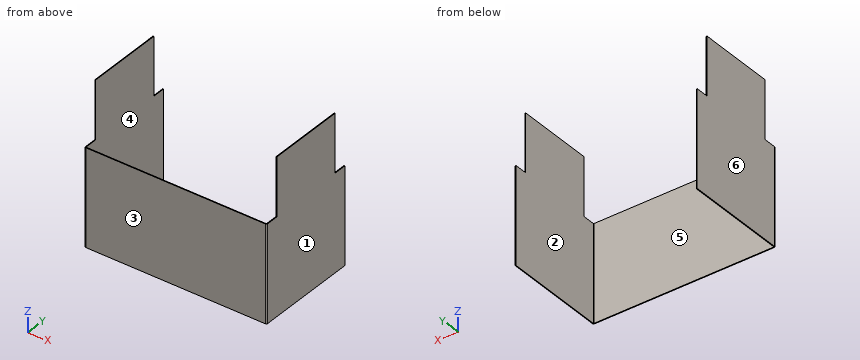
from build123d import *

# Parameters (mm, degrees)
SKETCH1_W                      = 317.5
SKETCH1_H                      = 1.5875
BASE_FLANGE1_DEPTH             = 355.6
EDGE_FLANGE1_STRIP_W           = 7.8232
EDGE_FLANGE1_STRIP_H           = 1.5875
EDGE_FLANGE1_STRIP_CUT_DEPTH   = 317.5
EDGE_FLANGE1_STRIP_2_W         = 7.8232
EDGE_FLANGE1_STRIP_2_H         = 1.5875
EDGE_FLANGE1_STRIP_CUT_2_DEPTH = 317.5
EDGE_FLANGE1_DEPTH             = 317.5
EDGE_FLANGE1_BEND_DEPTH        = 317.5
SKETCH8_W                      = 114.3
SKETCH8_H                      = 152.4
BOSS_EXTRUDE1_DEPTH            = 1.5875
SKETCH10_W                     = 127
SKETCH10_H                     = 254
CUT_EXTRUDE1_DEPTH             = 598.585693253


# Sheet-metal steps are written as plain solids
with BuildPart() as part:
    # Sketch1 → Base-Flange1 (new body)
    with BuildSketch(Plane(origin=(0, 0, 0), x_dir=(0, 0, -1), z_dir=(1, 0, 0))):
        with Locations((-158.75, 0.79375)):
            Rectangle(SKETCH1_W, SKETCH1_H)
    extrude(amount=BASE_FLANGE1_DEPTH)

    # Edge-Flange1 strip (across the edge) → Edge-Flange1 strip cut (cut)
    with BuildSketch(Plane(origin=(355.6, 1.5875, 317.5), x_dir=(-1, 0, 0), z_dir=(0, 0, -1))):
        with Locations((-3.175, -0.79375)):
            Rectangle(EDGE_FLANGE1_STRIP_W, EDGE_FLANGE1_STRIP_H)
    extrude(amount=EDGE_FLANGE1_STRIP_CUT_DEPTH, mode=Mode.SUBTRACT)

    # Edge-Flange1 strip 2 (across the edge) → Edge-Flange1 strip cut 2 (cut)
    with BuildSketch(Plane(origin=(0, 1.5875, 0), x_dir=(1, 0, 0), z_dir=(0, 0, 1))):
        with Locations((-3.175, -0.79375)):
            Rectangle(EDGE_FLANGE1_STRIP_2_W, EDGE_FLANGE1_STRIP_2_H)
    extrude(amount=EDGE_FLANGE1_STRIP_CUT_2_DEPTH, mode=Mode.SUBTRACT)

    # Edge-Flange1 section (across the edge) → Edge-Flange1 (add)
    with BuildSketch(Plane(origin=(355.6, 1.5875, 317.5), x_dir=(-1, 0, 0), z_dir=(0, 0, -1))):
        with BuildLine():
            Line((-1.5875, 0.7366), (-1.5875, 203.2))
            Line((-1.5875, 203.2), (0, 203.2))
            Line((0, 203.2), (0, 0.7366))
            ThreePointArc((0, 0.7366), (0.215745145, 0.215745145), (0.7366, 0))
            Line((0.7366, 0), (0.7366, -1.5875))
            ThreePointArc((0.7366, -1.5875), (-0.90678687, -0.90678687), (-1.5875, 0.7366))
        make_face()
    extrude(amount=EDGE_FLANGE1_DEPTH)

    # Edge-Flange1 section 2 (across the edge) → Edge-Flange1 bend (add)
    with BuildSketch(Plane(origin=(0, 1.5875, 0), x_dir=(1, 0, 0), z_dir=(0, 0, 1))):
        with BuildLine():
            Line((-1.5875, 0.7366), (-1.5875, 203.2))
            Line((-1.5875, 203.2), (0, 203.2))
            Line((0, 203.2), (0, 0.7366))
            ThreePointArc((0, 0.7366), (0.215745145, 0.215745145), (0.7366, 0))
            Line((0.7366, 0), (0.7366, -1.5875))
            ThreePointArc((0.7366, -1.5875), (-0.90678687, -0.90678687), (-1.5875, 0.7366))
        make_face()
    extrude(amount=EDGE_FLANGE1_BEND_DEPTH)


with BuildPart() as body_2:
    # Sketch8 → Boss-Extrude1 (new body)
    with BuildSketch(Plane(origin=(357.1875, 0, 0), x_dir=(0, 0, -1), z_dir=(1, 0, 0))):
        with Locations((-374.65, 103.1875)):
            Rectangle(SKETCH8_W, SKETCH8_H)
    extrude(amount=-BOSS_EXTRUDE1_DEPTH)


with BuildPart() as body_3:
    # Mirror1: mirrored copy
    add(body_2.part.mirror(Plane(origin=(177.8, 0, 0), x_dir=(0, 0, 1), z_dir=(1, 0, 0))))


with BuildPart() as body_2_1:
    add(body_2.part)

    # Combine1: union part, body 3
    add(part.part)
    add(body_3.part)

    # Sketch10 → Cut-Extrude1 (cut, through all)
    with BuildSketch(Plane(origin=(357.1875, 0, 0), x_dir=(0, 0, -1), z_dir=(1, 0, 0))):
        with Locations((-63.5, 77.7875)):
            Rectangle(SKETCH10_W, SKETCH10_H)
    extrude(amount=-CUT_EXTRUDE1_DEPTH, mode=Mode.SUBTRACT)


solid = body_2_1.part
Verification items for the finished model (mm, model axes). Face numbers are marked on the shaded views. A direction names the side the tool comes from. Coordinates: 2 decimals unless noted, no trailing zeros. Order: outer loops, then holes, each group sorted by start corner. A loop starts at its lowest first (then second) coordinate and runs counter-clockwise, first axis right, second up.
Item 1: Depth check by flat-ended pin: pin 1 (21.5 mm diameter, centred on x = 181.5, y = 13, fed in from +Z); pin 2 (1 mm diameter, centred on x = 241.5, z = 238, fed in from +Y); pin 3 (1.7 mm diameter, centred on x = -0.5, z = 374.5, fed in from +Y); pin 4 (1.7 mm diameter, centred on x = 357, z = 370.5, fed in from -Y). Enter the tip coordinate at first touch or a pass-through.
Filled in:
pin 1: passes through
pin 2: stops at y = 1.59
pin 3: stops at y = 179.39
pin 4: stops at y = 26.99
Item 2: Release check for a two-part mould opening along X. For the marked faces 1, 2, 3 and 4 record: +X half, -X half, draft (parallel to the pull), parting line (faces both ways), or undercut.
Filled in:
face 1: +X half
face 2: undercut
face 3: draft
face 4: undercut
Item 3: Access from +Z, -Z, +X, -X, +Y, -Y to the whole of each face (thin tool, end or side, straight path). Record for the marked faces 5 and 6.
Filled in:
face 5: +Z, -Z, +Y
face 6: +Z, -Z, -X, +Y, -Y
Item 4: Section check C-C, the plane z = 291. Enter the section's corners in (x, y), then the cut area to 3 significant figures.
Filled in:
outline: (-1.59, 2.32) arc R2.32 ccw to (0.74, 0) - (354.86, 0) arc R2.32 ccw to (357.19, 2.32) - (357.19, 204.79) - (355.6, 204.79) - (355.6, 2.32) arc R0.74 cw to (354.86, 1.59) - (0.74, 1.59) arc R0.74 cw to (0, 2.32) - (0, 204.79) - (-1.59, 204.79) - close
area: 1,210 mm2
Item 5: Section check B-B, the plane y = 115.5. Enter the section's corners in (x, z).
Filled in:
outline: (-1.59, 127) - (0, 127) - (0, 431.8) - (-1.59, 431.8) - close; (355.6, 127) - (357.19, 127) - (357.19, 431.8) - (355.6, 431.8) - close
Item 6: Section check D-D, the plane x = 259.5. Enter the section's corners in (y, z), then the cut area to 3 significant figures.
Filled in:
outline: (0, 127) - (1.59, 127) - (1.59, 317.5) - (0, 317.5) - close
area: 302 mm2
Item 7: Section check A-A, the plane z = 406.5. Enter the section's corners in (x, y), then the cut area to 3 significant figures.
Filled in:
outline: (-1.59, 26.99) - (0, 26.99) - (0, 179.39) - (-1.59, 179.39) - close; (355.6, 26.99) - (357.19, 26.99) - (357.19, 179.39) - (355.6, 179.39) - close
area: 484 mm2
Item 8: Material ranges on L1, parallel to X at y = 100, z = 152.5; L2, parallel to Y at x = 77, z = 143.5, recorded low to high.
Filled in:
L1: x = -1.59 to 0, 355.6 to 357.19
L2: y = 0 to 1.59
